Here's how the part is built. I have some questions about the finished solid (model axes, mm). A direction names the side the tool comes from. Round coordinates to 2 decimals unless told otherwise and drop trailing zeros. Write each loop counter-clockwise with the first axis right and the second up, starting at its lowest first coordinate (ties: lowest second). Pieces come first, ordered by that corner, then holes. Notation, with made-up numbers: M 40,5.25 L 47,5.25 A25 cw 47,32.25 Z; hole C 87.5,59 d6. An arc over 180 degrees is marked long. Use one line per item in the form item = value. Start each with the question number.
Q1. For faces 4 (the face through (-4, 0, 0)), 5 (the face through (280, 0, 0)), 6 (the face through (-267.298, 7, 5)), which set-ups out of +Z, -Z, +X, -X, +Y, -Y let a thin tool reach every point of the face, with its end or its side?
Q2. I want a section at A-A on z = 5. State how many separate pieces and enclosed holes the cut face has, and give its area (3 significant figures).
Q3. We'd pull the mould along X, two halves only. Please class faces 1 (the face through (267.298, 7, 5)), 2 (the face through (296.99, 7.15, 5.07)), 3 (the face through (280, 0, 10)): +X half, -X half, draft (parallel to the pull), parting line (faces both ways), or undercut.
Q4. I want a section at B-B on x = -257.5. List the corners of the cut face in (y, z) for me.
Q5. I need wall thicknesses on line 1 along X through (y, z) = (-1, 5.75); line 2 along X through (y, z) = (-7.25, 1.5); line 3 along Y through (x, z) = (-290, 5.5). Which ranges of each line are inside material? Lowest first, please. Write a range as from..to.
Q6. I'm going to push flat-ended pins straight in: pin 1 Ø1.5 at (x, z) = (93, 1.5) entering from -Y; pin 2 Ø4 at (x, y) = (-132, 3) entering from -Z; pin 3 Ø2 at (x, y) = (94, 3) entering from -Z. Where does each tip first touch, or does it pass through?
```python
from build123d import *

# Parameters (mm, degrees)
SKETCH_1_W          = 600
SKETCH_1_H          = 20
SKETCH_1_R          = 7
EXTRUDE_1_DEPTH     = 10
FILLET_1_R          = 10
SKETCH1_W           = 534.59629528
SKETCH1_H           = 41.86621972
CUT_EXTRUDE1_DEPTH  = 19
SKETCH2_R           = 5
BOSS_EXTRUDE1_DEPTH = 535


with BuildPart() as part:
    # 草图1 → 凸台-拉伸1 (new body)
    with BuildSketch(Plane.XY):
        Rectangle(SKETCH_1_W, SKETCH_1_H)
        with Locations((-290, 0)):
            Circle(SKETCH_1_R, mode=Mode.SUBTRACT)
        with Locations((290, 0)):
            Circle(SKETCH_1_R, mode=Mode.SUBTRACT)
    extrude(amount=EXTRUDE_1_DEPTH)

    # 圆角1
    fillet_1_edges = [part.edges().sort_by_distance(p)[0] for p in [
        (300, 10, 5),
        (300, -10, 5),
        (-300, -10, 5),
        (-300, 10, 5),
    ]]
    fillet(fillet_1_edges, radius=FILLET_1_R - 0.0001)  # a hair under: the kernel refuses the full size

    # Sketch1 → Cut-Extrude1 (cut)
    with BuildSketch(Plane.XY):
        Rectangle(SKETCH1_W, SKETCH1_H)
    extrude(amount=CUT_EXTRUDE1_DEPTH, mode=Mode.SUBTRACT)


with BuildPart() as cut_extrude1_piece_1:
    # of the separate pieces the step leaves, piece 1, a body of its own (cut_extrude1_pieces)
    add(part.part.solids().sort_by_distance((-290.0001, -10, 0))[0])



with BuildPart() as cut_extrude1_piece_2:
    # of the separate pieces the step leaves, piece 2, a body of its own (cut_extrude1_pieces)
    add(part.part.solids().sort_by_distance((267.29814764, -10, 0))[0])


with BuildPart() as cut_extrude1_piece_1_1:
    add(cut_extrude1_piece_1.part)

    add(cut_extrude1_piece_2.part)  # Boss-Extrude1 merges Cut-Extrude1 piece 2
    # Sketch2 → Boss-Extrude1 (add)
    with BuildSketch(Plane(origin=(-267.29814764, 0, 0), x_dir=(0, 0, -1), z_dir=(1, 0, 0))):
        with Locations(Location((-5, 0, 0), (0, 0, 180))):
            Circle(SKETCH2_R)
    extrude(amount=BOSS_EXTRUDE1_DEPTH)


solid = cut_extrude1_piece_1_1.part
```
Reported:
q1.face_4 = none
q1.face_5 = -Z, +X, -X, +Y, -Y
q1.face_6 = +Y
q2.separate_pieces = 1
q2.enclosed_holes = 2
q2.area = 6,260 mm^2
q3.face_1 = undercut
q3.face_2 = +X half
q3.face_3 = draft
q4.outline = C 0,5 d10
q5.line_1 = -299.95..-296.93, -283.07..283.07, 296.93..299.95
q5.line_2 = -296.89..-267.3, 267.3..296.89
q5.line_3 = -10..-7, 7..10
q6.pin_1 = -4.18
q6.pin_2 = 0.1
q6.pin_3 = 0.42
